from build123d import *

# Parameters (mm, degrees)
BOSS_EXTRUDE1_DEPTH = 22.225
SKETCH2_W           = 95.09357109
SKETCH2_H           = 14.776094164
BOSS_EXTRUDE2_DEPTH = 11.1125
SKETCH3_W           = 105.533171411
SKETCH3_H           = 8.318821745
CUT_EXTRUDE1_DEPTH  = 6.35
CUT_EXTRUDE2_DEPTH  = 444.471216787
BOSS_EXTRUDE3_DEPTH = 11.1125
CHAMFER1_SIZE       = 3.175


with BuildPart() as part:
    # Sketch1 → Boss-Extrude1 (new body)
    with BuildSketch(Plane.XY):
        Polygon((219.382736593, 187.272406651), (219.382736593, 231.378695124), (252.047484341, 257.668279987), (286.011346283, 257.668279987), (286.011346283, 253.335489362), (340.095731947, 253.335489362), (340.095731947, 257.668279987), (340.095731947, 262.071092462), (355.810019244, 262.071092462), (357.059535637, 164.129151492), (345.471646064, 164.129151492), (345.471646064, 189.97898492), (250.378074974, 189.97898492), (282.230145695, 168.148416333), (247.35103376, 168.148416333), align=None)
    extrude(amount=BOSS_EXTRUDE1_DEPTH)

    # Sketch2 → Boss-Extrude2 (add)
    with BuildSketch(Plane.XY):
        with Locations((297.924860519, 182.590937838)):
            Rectangle(SKETCH2_W, SKETCH2_H)
    extrude(amount=BOSS_EXTRUDE2_DEPTH)

    # Sketch3 → Cut-Extrude1 (cut)
    with BuildSketch(Plane.XY.offset(22.225)):
        with Locations((272.149322299, 212.351794066)):
            Rectangle(SKETCH3_W, SKETCH3_H)
        Polygon((340.095731947, 253.335489362), (340.095731947, 234.12753334), (252.166996271, 234.12753334), (286.011346283, 257.668279987), align=None)
    extrude(amount=-CUT_EXTRUDE1_DEPTH, mode=Mode.SUBTRACT)

    # Sketch4 → Cut-Extrude2 (cut, through all)
    with BuildSketch(Plane.XY.offset(22.225)):
        with BuildLine():
            Line((232.799757397, 227.389091829), (340.459546105, 227.389091829))
            ThreePointArc((340.459546105, 227.389091829), (343.600105184, 224.24853275), (340.459546105, 221.107973671))
            Line((340.459546105, 221.107973671), (232.799757397, 221.107973671))
            ThreePointArc((232.799757397, 221.107973671), (229.659198318, 224.24853275), (232.799757397, 227.389091829))
        make_face()
        with BuildLine():
            Line((232.771208039, 203.900524193), (340.426548272, 204.879209104))
            ThreePointArc((340.426548272, 204.879209104), (343.595526941, 201.76732915), (340.483646987, 198.598350481))
            Line((340.483646987, 198.598350481), (232.828306754, 197.619665569))
            ThreePointArc((232.828306754, 197.619665569), (229.659328085, 200.731545524), (232.771208039, 203.900524193))
        make_face()
    extrude(amount=-CUT_EXTRUDE2_DEPTH, mode=Mode.SUBTRACT)

    # Sketch5 → Boss-Extrude3 (add)
    with BuildSketch(Plane.XY.offset(11.1125)):
        Polygon((282.230145695, 168.148416333), (282.230145695, 175.202890756), (271.937256742, 175.202890756), align=None)
    extrude(amount=-BOSS_EXTRUDE3_DEPTH)

    # Chamfer1
    chamfer1_edges = [part.edges().sort_by_distance(p)[0] for p in [
        (340.095731947, 248.099312901, 22.225),
        (345.471646064, 177.054068206, 22.225),
        (266.304110334, 179.063700626, 22.225),
        (269.089171277, 245.897906663, 22.225),
    ]]
    chamfer(chamfer1_edges, length=CHAMFER1_SIZE)


solid = part.part
For this review, take the finished solid that the model builds, in its own axes (mm). A direction names the side the tool comes from. Round coordinates to 2 decimals unless told otherwise and drop trailing zeros. Loops run counter-clockwise (first coordinate to the right, second up) from the corner with the lowest first, then second, coordinate; pieces in that order, holes last. Notation, with made-up numbers: (-10, 22) - (4, 22) arc R17 cw to (4, 26) - close; hole circle Ø2 at (76.25, 38.5). An arc over 180 degrees is marked (long way). Use one line per item in the form item = value.
Item 1: Consider section C-C on y = 200. Write out the cut boundary in (x, z) (3 decimals), then the cut area to 3 significant figures.
Answers:
outline = (219.383, 0) - (229.753, 0) - (229.753, 22.225) - (219.383, 22.225) - close; (343.07, 0) - (356.602, 0) - (356.602, 22.225) - (343.07, 22.225) - close
area = 531 mm^2
Item 2: Tool access review of faces 4 (the flat face through (345.472, 174, 12)), 5 (the flat face through (341.661, 247.904, 20.615)), 6 (the flat face through (313, 253.335, 8)), 7 (the cylindrical face through (229.66, 224.18, 11.27)): name each direction out of +Z, -Z, +X, -X, +Y, -Y from which nothing blocks a thin tool from reaching the whole face with its end or side.
Answers:
face_4 = +Z, -Y
face_5 = +Z, +Y
face_6 = +Z, -Z, +Y
face_7 = +Z, -Z
Item 3: Consider section A-A on z = 6.5. Write out the cut boundary in (x, y).
Answers:
outline = (219.38, 187.27) - (247.35, 168.15) - (282.23, 168.15) - (282.23, 175.2) - (345.47, 175.2) - (345.47, 164.13) - (357.06, 164.13) - (355.81, 262.07) - (340.1, 262.07) - (340.1, 253.34) - (286.01, 253.34) - (286.01, 257.67) - (252.05, 257.67) - (219.38, 231.38) - close; hole (232.77, 203.9) arc R3.14 ccw to (232.83, 197.62) - (340.48, 198.6) arc R3.14 ccw to (340.43, 204.88) - close; hole (232.8, 221.11) - (340.46, 221.11) arc R3.14 ccw to (340.46, 227.39) - (232.8, 227.39) arc R3.14 ccw to start
Item 4: Clearance check with flat-ended pins moving along their axes: P1, Ø5, axis at y = 250, z = 17.5, coming from the -X side; P2, Ø1.9, axis at x = 312.5, z = 19, coming from the +Y side; P3, Ø5, axis at y = 256.5, z = 7, coming from the +X side. State where each tip first meets the part, or that it passes through.
Answers:
P1 = 239.41
P2 = 234.13
P3 = 355.91
Item 5: Consider section D-D on z = 12.75. Write out the cut boundary in (x, y), then the cut area to 3 significant figures.
Answers:
outline = (219.38, 187.27) - (247.35, 168.15) - (282.23, 168.15) - (250.38, 189.98) - (345.47, 189.98) - (345.47, 164.13) - (357.06, 164.13) - (355.81, 262.07) - (340.1, 262.07) - (340.1, 253.34) - (286.01, 253.34) - (286.01, 257.67) - (252.05, 257.67) - (219.38, 231.38) - close; hole (232.77, 203.9) arc R3.14 ccw to (232.83, 197.62) - (340.48, 198.6) arc R3.14 ccw to (340.43, 204.88) - close; hole (232.8, 221.11) - (340.46, 221.11) arc R3.14 ccw to (340.46, 227.39) - (232.8, 227.39) arc R3.14 ccw to start
area = 8,310 mm^2
Item 6: Mouldability with a two-part tool opening along X and no side actions: class faces 1 (the flat face through (233.56, 177.58, 10.96)), 2 (the flat face through (286, 227.389, 11)), 3 (the flat face through (269, 257.668, 11)) as +X half, -X half, draft (parallel to the pull), parting line (faces both ways), or undercut.
Answers:
face_1 = -X half
face_2 = undercut
face_3 = draft
Item 7: For line 1 (Y direction, x = 326, z = 10); line 2 (Y direction, x = 260.5, z = 16.5); line 3 (Y direction, x = 298, z = 4.75), list the stretches that pass through material, from the lowest coordinate up.
Answers:
line_1 = 175.2 to 198.47, 204.75 to 221.11, 227.39 to 253.34
line_2 = 168.15 to 183.04, 189.98 to 197.87, 204.15 to 208.19, 216.51 to 221.11, 227.39 to 234.13, 239.92 to 257.67
line_3 = 175.2 to 198.21, 204.49 to 221.11, 227.39 to 253.34
Item 8: Consider section B-B on x = 262. State how many separate pieces and enclosed holes the cut face has, then the cut area to 3 significant figures.
Answers:
separate_pieces = 3
enclosed_holes = 0
area = 1,510 mm^2
